from build123d import *

# Parameters (mm, degrees)
F0_W     = 6.35
F0_H     = 12.1919997036
F0_H_2   = 35.5785874814
F0_W_2   = 12.1919997036
F0_H_3   = 6.35
F1_DEPTH = 25.4


with BuildPart() as f1:
    # F0 (on Top) → F1 (new body)
    with BuildSketch(Plane.XY):
        with Locations((-33.7727085769, -23.6963424832)):
            Rectangle(F0_W, F0_H)
        Polygon((-30.5977085769, -17.6003426313), (-30.5977085769, -29.792342335), (44.2331731319, -29.792342335), (44.2331731319, 17.97824485), (32.0411734283, 17.97824485), (32.0411734283, -17.6003426313), align=None)
        with Locations((-33.7727085769, 0.1889511093)):
            Rectangle(F0_W, F0_H_2)
        Polygon((-36.9477085769, 24.32824485), (-36.9477085769, 17.97824485), (-30.5977085769, 17.97824485), (-30.5977085769, 20.4689776353), align=None)
        with Locations((38.1371732801, 21.15324485)):
            Rectangle(F0_W_2, F0_H_3)
        Polygon((-30.5977085769, 24.32824485), (-36.9477085769, 24.32824485), (-30.5977085769, 20.4689776353), align=None)
        Polygon((-26.4994815545, 17.97824485), (32.0411734283, 17.97824485), (32.0411734283, 24.32824485), (-30.5977085769, 24.32824485), (-30.5977085769, 20.4689776353), align=None)
    extrude(amount=F1_DEPTH)


solid = f1.part
The model under review builds one solid part; all positions refer to its coordinate system, in mm. A direction names the side the tool comes from. Round coordinates to 2 decimals unless told otherwise and drop trailing zeros. Write each loop counter-clockwise with the first axis right and the second up, starting at its lowest first coordinate (ties: lowest second). Pieces come first, ordered by that corner, then holes. Notation, with made-up numbers: M 40,82.25 L 71,82.25 A8 cw 71,87.25 Z; hole C 19.25,20 d4. An arc over 180 degrees is marked long. Use a Markdown table: item, result. Add a question column.
Q1. We need section C-C, the plane z = 9.25. State the section outline as (x, y) points.
Q2. We need section A-A, the plane y = -3.5. State the section outline as (x, z) points, plus the area to 3 significant figures.
Q3. To check wall thickness, follow line 1 (Y direction, x = 26.5, z = 23.75); line 2 (X direction, y = 12.5, z = 9.5); line 3 (X direction, y = 18.5, z = 8). State the ranges of each line that lie inside material, in increasing order.
Q4. We need section B-B, the plane x = -6. State the section outline as (y, z) points.
Q5. Machinability: for faces 1 (the face through (3, -20, 25.4)), 2 (the face through (-30.598, 1, 13)), which of the approach directions +Z, -Z, +X, -X, +Y, -Y give a long, thin tool a straight path to every point of the face, cutting with its end or side? Answer none if there is none.
Q6. The part is to be moulded in two halves that separate along X. For faces 3 (the face through (44.233, -3, 13)), 4 (the face through (1, -17.6, 13)), 5 (the face through (3, -20, 0)), 6 (the face through (-36.948, -2, 13)), say which applies: pulls with the +X half, pulls with the -X half, needs draft (parallel to the pull), parting line crosses it, or undercut.
Findings below:
| question | item | result |
|---|---|---|
| 1 | outline | M -36.95,-29.79 L 44.23,-29.79 L 44.23,24.33 L -36.95,24.33 Z; hole M -30.6,-17.6 L 32.04,-17.6 L 32.04,17.98 L -26.5,17.98 L -30.6,20.47 Z |
| 2 | outline | M -36.95,0 L -30.6,0 L -30.6,25.4 L -36.95,25.4 Z; M 32.04,0 L 44.23,0 L 44.23,25.4 L 32.04,25.4 Z |
| 2 | area | 471 mm² |
| 3 | line 1 | y = -29.79 to -17.6, 17.98 to 24.33 |
| 3 | line 2 | x = -36.95 to -30.6, 32.04 to 44.23 |
| 3 | line 3 | x = -36.95 to -30.6, -27.36 to 44.23 |
| 4 | outline | M -29.79,0 L -17.6,0 L -17.6,25.4 L -29.79,25.4 Z; M 17.98,0 L 24.33,0 L 24.33,25.4 L 17.98,25.4 Z |
| 5 | face 1 | +Z, +X, -X, +Y, -Y |
| 5 | face 2 | +Z, -Z |
| 6 | face 3 | pulls with the +X half |
| 6 | face 4 | undercut |
| 6 | face 5 | needs draft |
| 6 | face 6 | pulls with the -X half |
